Part model, mm, in its own coordinate system. Face numbers are marked on the shaded views. A direction names the side the tool comes from. Round coordinates to 2 decimals unless told otherwise and drop trailing zeros. Loops run counter-clockwise (first coordinate to the right, second up) from the corner with the lowest first, then second, coordinate; pieces in that order, holes last. Notation, with made-up numbers: (81, -22) - (123, -22) arc R24 ccw to (123, 8) - close; hole circle Ø2 at (83, 32). An arc over 180 degrees is marked (long way). Put each result on its own line as item: value.
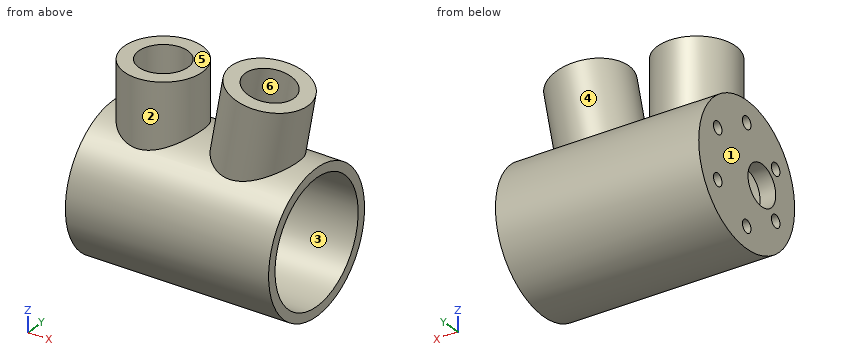
Autodesk Inventor part; units mm, degrees
ref_plane "Work Plane1" through (0, 0, 40) normal (0, 0, 1) x (1, 0, 0)
ref_plane "Work Plane2" through (32.5, -22.5, 40) normal (0.1736, 0, 0.9848) x (0, 1, 0)
ref_plane "YZ Plane" through (0, 0, 0) normal (1, 0, 0) x (0, 1, 0)
sketch "Sketch2" plane through (0, 0, 0) normal (1, 0, 0) x (0, 1, 0)
  circle A0 centre (0, 0) radius 19.5
  circle A1 centre (0, 0) radius 22.5
  dimension "d0" = 39
  dimension "d1" = 45
extrude "Extrusion1" add sketch "Sketch2" along normal mid plane 65 contours A0 | A1
sketch "Sketch3" plane through (32.5, 0, 0) normal (1, 0, 0) x (0, 0, -1)
  circle A0 centre (0, 0) radius 19.5
  dimension "d4" = 39
extrude "Extrusion2" cut sketch "Sketch3" against normal blind 60
sketch "Sketch4" plane through (-32.5, 0, 0) normal (-1, 0, 0) x (0, 0, 1)
  circle A0 centre (-15.7, 0) radius 2
  point P0 (0, 0)
  point P1 (0, 0)
  dimension "d7" = 4
  dimension "d45" = 15.7
extrude "Extrusion3" cut sketch "Sketch4" against normal blind 5
pattern_circular "Circular Pattern1" count 6 over 360 about axis through (-10, 0, 0) along (1, 0, 0) of "Extrusion3"
sketch "Sketch5" plane through (-32.5, 0, 0) normal (-1, 0, 0) x (0, 0, 1)
  circle A0 centre (0, -7.11) radius 6.5
  point P0 (0, 0)
  dimension "d13" = 13
extrude "Extrusion4" cut sketch "Sketch5" against normal blind 5
ref_plane "Work Plane1" through (0, 0, 40) normal (0, 0, 1) x (1, 0, 0)
sketch "Sketch6" plane through (0, 0, 40) normal (0, 0, 1) x (1, 0, 0)
  circle A0 centre (-16.4979, 0) radius 12.5
  circle A1 centre (-16.4979, 0) radius 7.9
  point P0 (0, 0)
  dimension "d17" = 25
  dimension "d18" = 15.8
extrude "Extrusion5" add sketch "Sketch6" against normal up to surface
sketch "Sketch7" plane through (0, 0, 40) normal (0, 0, 1) x (1, 0, 0)
  line L0 (32.5, -22.5) -> (32.5, 22.5)
  point P0 (0, 0)
ref_plane "Work Plane2" through (32.5, -22.5, 40) normal (0.1736, 0, 0.9848) x (0, 1, 0)
sketch "Sketch8" plane through (32.5, -22.5, 40) normal (0.1736, 0, 0.9848) x (0, 1, 0)
  circle A0 centre (22.5, 15.2535) radius 12.5
  circle A1 centre (22.5, 15.2535) radius 7.9
  ellipse E0 centre (22.5, 48.2535) end of major axis (30.4, 48.2535) minor radius 7.78
  point P0 (22.5, 25.0603)
  dimension "d22" = 25
  dimension "d23" = 15.8
  dimension "d26" = 33
extrude "Extrusion6" add sketch "Sketch8" against normal up to surface contours A0
sketch "Sketch9" plane through (-32.5, 0, 0) normal (-1, 0, 0) x (0, 0, 1)
  circle A0 centre (0, -7.11) radius 6.5
  circle A1 centre (-7.85, -13.5966) radius 2
  circle A2 centre (7.85, -13.5966) radius 2
  circle A3 centre (15.7, 0) radius 2
  circle A4 centre (7.85, 13.5966) radius 2
  circle A5 centre (-7.85, 13.5966) radius 2
  circle A6 centre (-15.7, 0) radius 2
  circle A7 centre (0, 0) radius 22.5
properties part number "SoporteMotor" material "PLA"
1. Band-saw the part on C-C (x = -19.5). List the corners of the cut face in (y, z), plus the area to 3 significant figures.
A:
outline: (-12.13, 18.95) arc R22.5 ccw (long way) to (12.13, 18.95) - (12.13, 40) - (7.31, 40) - (7.31, 21.28) arc R22.5 ccw to (-7.31, 21.28) - (-7.31, 40) - (-12.13, 40) - close; hole circle Ø39 at (0, 0)
area: 587 mm²
2. Tool access for the marked faces 1 and 2: list every direction of +Z, -Z, +X, -X, +Y, -Y with a clear straight run to the whole face (end or side of a thin tool).
A:
face 1: +Z, -Z, -X, +Y, -Y
face 2: +Z
3. Band-saw the part on A-A (z = 8). List the corners of the cut face in (x, y).
A:
outline: (-32.5, -21.03) - (32.5, -21.03) - (32.5, -17.78) - (-27.5, -17.78) - (-27.5, -15.59) - (-32.5, -15.59) - close; (-32.5, -11.6) - (-27.5, -11.6) - (-27.5, 11.6) - (-32.5, 11.6) - close; (-32.5, 15.59) - (-27.5, 15.59) - (-27.5, 17.78) - (32.5, 17.78) - (32.5, 21.03) - (-32.5, 21.03) - close
4. Band-saw the part on D-D (z = 15.7). List the corners of the cut face in (x, y).
A:
outline: (-32.5, -16.12) - (32.5, -16.12) - (32.5, -11.57) - (-27.5, -11.57) - (-27.5, -2) - (-32.5, -2) - close; (-32.5, 2) - (-27.5, 2) - (-27.5, 11.57) - (32.5, 11.57) - (32.5, 16.12) - (-32.5, 16.12) - close
5. Band-saw the part on B-B (y = 18.5). List the corners of the cut face in (x, z).
A:
outline: (-32.5, -12.81) - (32.5, -12.81) - (32.5, -6.16) - (-27.5, -6.16) - (-27.5, 6.16) - (32.5, 6.16) - (32.5, 12.81) - (-32.5, 12.81) - close
6. Two-plate mould, pull along Y, no slides. Class the marked faces 3, 4, 5 and 6: pulls with the +Y half, pulls with the -Y half, needs draft (parallel to the pull), parting line crosses it, or undercut.
A:
face 3: undercut
face 4: parting line crosses it
face 5: needs draft
face 6: undercut
7. Pin check, flat tips, straight feed: P1, Ø1, axis at y = 9, z = 27, coming from the +X side; P2, Ø10, axis at x = 18.5, z = 30.5, coming from the +Y side; P3, Ø4.5, axis at y = 0, z = 15.7, coming from the -X side; P4, Ø5, axis at x = -1.5, y = 6, coming from the -Z side. Stop position of each tip, or through.
A:
P1: stops at x = 24.03
P2: stops at y = 12.5
P3: stops at x = -32.5
P4: stops at z = -22.23
8. Probe line 1 along X through (y, z) = (0, 30); line 2 along X through (y, z) = (8.5, -3.5); line 3 along Z through (x, y) = (0.5, 17). List the from-to ranges inside material, lowest first. Write a range as [from, to].
A:
line 1: x = [-29, -24.4], [-8.6, -4], [2.56, 7.23], [23.27, 27.94]
line 2: x = [-32.5, -27.5]
line 3: z = [-14.74, -9.55], [9.55, 14.74]
